Autodesk Inventor part; units mm, degrees
ref_plane "Work Plane1" through (0, 0, -3) normal (0, 0, 1) x (1, 0, 0)
ref_plane "YZ Plane" through (0, 0, 0) normal (1, 0, 0) x (0, 1, 0)
ref_plane "XZ Plane" through (0, 0, 0) normal (0, 1, 0) x (-1, 0, 0)
ref_plane "Work Plane1" through (0, 0, -3) normal (0, 0, 1) x (1, 0, 0)
sketch "Sketch1" plane through (0, 0, -3) normal (0, 0, 1) x (1, 0, 0)
  circle A0 centre (0, 0) radius 2.75
extrude "Extrusion3" add sketch "Sketch1" along normal blind 3
fillet "Fillet1" radius 0.1 2 edges at (-2.75, 0, -3) (-2.75, 0, 0)
sketch "Sketch2" plane through (0, 0, -3) normal (0, 0, 1) x (1, 0, 0)
  line L0 (-0.7217, 1.25) -> (0.7217, 1.25)
  line L1 (0.7217, -1.25) -> (-0.7217, -1.25)
  line L2 (-0.7217, -1.25) -> (-1.4434, 0)
  line L3 (0.7217, 1.25) -> (1.4434, 0)
  line L4 (-1.4434, 0) -> (-0.7217, 1.25)
  line L5 (1.4434, 0) -> (0.7217, -1.25)
extrude "Extrusion2" cut sketch "Sketch2" along normal blind 3
sketch "Sketch3" plane through (0, 0, 0) normal (0, 0, 1) x (1, 0, 0)
  circle A0 centre (0, 0) radius 1.5
extrude "Extrusion1" add sketch "Sketch3" along normal blind 4
chamfer "Chamfer1" distance 0.2 angle 45 1 edges at (-1.5, 0, 4)
properties part number "M3 x 4mm SHCS" material "Stainless Steel"
Can you work these out from the model? Positions are in its coordinate system, mm. A direction names the side the tool comes from. Give positions to 0.01 mm unless a question says otherwise; leave off trailing zeros. Write each loop counter-clockwise with the first axis right and the second up, starting at its lowest first coordinate (ties: lowest second). Pieces come first, ordered by that corner, then holes. Notation, with made-up numbers: (63, 76) -> (86, 76) arc R16 ccw to (86, 86) -> close; hole circle Ø3 at (62.25, 73). An arc over 180 degrees is marked (long way). Answer as a JSON object with one key per item and string values. Group by question number.
Item 1: Suppose I cut it at B-B (x = 0). Please give me the cut outline in (y, z), plus the area to 3 significant figures.
Item 2: I'm going to push a flat-ended pin straight in: P1, Ø1.5, axis at x = -2, z = 2, coming from the -Y side. Where does the tip first touch, or does it pass through?
Item 3: Please list where these lines run through material, in increasing order: line 1 (X direction, y = 1.1, z = -0.75); line 2 (X direction, y = 0.85, z = -1.5); line 3 (Z direction, x = 1.15, y = -0.3). Write a range as [from, to].
Item 4: Suppose I cut it at C-C (z = 0.25). Please give me the cut outline in (x, y).
Item 5: Suppose I cut it at A-A (z = -1.5). Please give me the cut outline in (x, y), plus the area to 3 significant figures.
Item 6: We'd pull the mould along X, two halves only. Please class faces 1 (the face through (-1.5, -0.07, 1.87)), 2 (the face through (1.08, 0.63, -1.52)), 3 (the face through (-1.08, -0.63, -1.52)), 4 (the face through (0, -2, 0)): +X half, -X half, draft (parallel to the pull), parting line (faces both ways), or undercut.
Item 7: For faces 5 (the face through (0, -1.25, -2)), 6 (the face through (0, 0, 4)), which set-ups out of +Z, -Z, +X, -X, +Y, -Y let a thin tool reach every point of the face, with its end or its side?
Findings:
{
 "1": {"outline": "(-2.75, -2.9) arc R0.1 ccw to (-2.65, -3) -> (-1.25, -3) -> (-1.25, 0) -> (1.25, 0) -> (1.25, -3) -> (2.65, -3) arc R0.1 ccw to (2.75, -2.9) -> (2.75, -0.1) arc R0.1 ccw to (2.65, 0) -> (1.5, 0) -> (1.5, 3.8) -> (1.3, 4) -> (-1.3, 4) -> (-1.5, 3.8) -> (-1.5, 0) -> (-2.65, 0) arc R0.1 ccw to (-2.75, -0.1) -> close", "area": "21.0 mm²"},
 "2": {"P1": "stops at y = -0.83"},
 "3": {"line 1": "x = [-2.52, -0.81], [0.81, 2.52]", "line 2": "x = [-2.62, -0.95], [0.95, 2.62]", "line 3": "z = [0, 4]"},
 "4": {"outline": "circle Ø3 at (0, 0)"},
 "5": {"outline": "circle Ø5.5 at (0, 0); hole (-1.44, 0) -> (-0.72, -1.25) -> (0.72, -1.25) -> (1.44, 0) -> (0.72, 1.25) -> (-0.72, 1.25) -> close", "area": "18.3 mm²"},
 "6": {"face 1": "parting line", "face 2": "undercut", "face 3": "undercut", "face 4": "draft"},
 "7": {"face 5": "-Z", "face 6": "+Z, +X, -X, +Y, -Y"}
}
